```python
from build123d import *

# Parameters (mm, degrees)
BOSS_EXTRUDE1_DEPTH = 3
SKETCH2_R           = 2
CUT_EXTRUDE1_DEPTH  = 3
SKETCH3_R           = 2.5
SKETCH3_R_2         = 2
BOSS_EXTRUDE2_DEPTH = 6


with BuildPart() as part:
    # Sketch1 → Boss-Extrude1 (new body)
    with BuildSketch(Plane.XY):
        Polygon((4, 0), (39, 0), (39, 38), (0, 38), (0, 27), (4, 27), align=None)
    extrude(amount=BOSS_EXTRUDE1_DEPTH)

    # Sketch2 → Cut-Extrude1 (cut)
    with BuildSketch(Plane.XY.offset(3)):
        with Locations((5.37, 31.4)):
            Circle(SKETCH2_R)
        with Locations((25.4, 31.4)):
            Circle(SKETCH2_R)
        with Locations((10.5, 5)):
            Circle(SKETCH2_R)
    extrude(amount=-CUT_EXTRUDE1_DEPTH, mode=Mode.SUBTRACT)

    # Sketch3 → Boss-Extrude2 (add)
    with BuildSketch(Plane.XY.offset(3)):
        with Locations((5.37, 31.4)):
            Circle(SKETCH3_R)
        with Locations((5.37, 31.4)):
            Circle(SKETCH3_R_2, mode=Mode.SUBTRACT)
        with Locations((25.4, 31.4)):
            Circle(SKETCH3_R)
        with Locations((25.4, 31.4)):
            Circle(SKETCH3_R_2, mode=Mode.SUBTRACT)
        with Locations((10.5, 5)):
            Circle(SKETCH3_R)
        with Locations((10.5, 5)):
            Circle(SKETCH3_R_2, mode=Mode.SUBTRACT)
    extrude(amount=-BOSS_EXTRUDE2_DEPTH)


solid = part.part
```
Verification items for the finished model (mm, model axes). A direction names the side the tool comes from. Round coordinates to 2 decimals unless told otherwise and drop trailing zeros. Write each loop counter-clockwise with the first axis right and the second up, starting at its lowest first coordinate (ties: lowest second). Pieces come first, ordered by that corner, then holes. Notation, with made-up numbers: (40, -7) -> (76, -7) arc R24 cw to (76, 27) -> close; hole circle Ø10 at (53.5, -36). An arc over 180 degrees is marked (long way). Write each question's results on one line, items separated by ' | '. Start each with the question number.
1. Cross-section at B-B (x = 5.37). Enter the section's corners in (y, z).
2. Cross-section at D-D (y = 31.4). Enter the section's corners in (x, z).
3. Material ranges on probe 1 along X at (y, z) = (31.5, 0.15); probe 2 along Y at (x, z) = (25.4, 0.35); probe 3 along Y at (x, z) = (5.37, -1.75), recorded low to high. Write a range as from..to.
4. Depth check by flat-ended pin: P1, Ø1, axis at x = 34.5, z = 1, coming from the -Y side; P2, Ø6, axis at x = 25, y = 13.5, coming from the -Z side; P3, Ø0.9, axis at x = 1.5, z = 1.5, coming from the -Y side; P4, Ø2.5, axis at y = 14.5, z = 2, coming from the -X side. Enter the tip coordinate at first touch or a pass-through.
5. Draft check along Y on faces 1 (the cylindrical face through (6.71, 33.51, -1.48)), 2 (the cylindrical face through (4.936, 29.448, 0.042)), 3 (the flat face through (4, 14, 1)). Enter one of: +Y half, -Y half, draft (parallel to the pull), parting line (faces both ways), or undercut.
6. Cross-section at A-A (y = 5). Enter the section's corners in (x, z), then the cut area to 3 significant figures.
7. Set-up check for faces 4 (the cylindrical face through (26.74, 33.51, -1.48)), 5 (the cylindrical face through (26.323, 29.626, 0.042)), 6 (the flat face through (2, 27, 1)): record each of +Z, -Z, +X, -X, +Y, -Y from which the full face is reachable in a straight line by a thin tool's end or side.
8. Cross-section at C-C (z = 1.7). Enter the section's corners in (x, y), then the cut area to 3 significant figures.
Solutions:
1) outline: (0, 0) -> (28.9, 0) -> (28.9, -3) -> (29.4, -3) -> (29.4, 3) -> (0, 3) -> close; (33.4, -3) -> (33.9, -3) -> (33.9, 0) -> (38, 0) -> (38, 3) -> (33.4, 3) -> close
2) outline: (0, 0) -> (2.87, 0) -> (2.87, -3) -> (3.37, -3) -> (3.37, 3) -> (0, 3) -> close; (7.37, -3) -> (7.87, -3) -> (7.87, 0) -> (22.9, 0) -> (22.9, -3) -> (23.4, -3) -> (23.4, 3) -> (7.37, 3) -> close; (27.4, -3) -> (27.9, -3) -> (27.9, 0) -> (39, 0) -> (39, 3) -> (27.4, 3) -> close
3) probe 1: x = 0..3.37, 7.37..23.4, 27.4..39 | probe 2: y = 0..29.4, 33.4..38 | probe 3: y = 28.9..29.4, 33.4..33.9
4) P1: stops at y = 0 | P2: stops at z = 0 | P3: stops at y = 27 | P4: stops at x = 4
5) face 1: parting line | face 2: undercut | face 3: draft
6) outline: (4, 0) -> (8, 0) -> (8, -3) -> (8.5, -3) -> (8.5, 3) -> (4, 3) -> close; (12.5, -3) -> (13, -3) -> (13, 0) -> (39, 0) -> (39, 3) -> (12.5, 3) -> close | area: 96.0 mm2
7) face 4: -Z | face 5: +Z, -Z | face 6: +Z, -Z, -X, -Y
8) outline: (0, 27) -> (4, 27) -> (4, 0) -> (39, 0) -> (39, 38) -> (0, 38) -> close; hole circle Ø4 at (5.37, 31.4); hole circle Ø4 at (10.5, 5); hole circle Ø4 at (25.4, 31.4) | area: 1,340 mm2
